from build123d import *

# Parameters (mm, degrees)
SKETCH1_W           = 50
SKETCH1_H           = 85
SKETCH1_R           = 1.25
BOSS_EXTRUDE3_DEPTH = 4
SKETCH2_W           = 50
SKETCH2_H           = 85
SKETCH2_W_2         = 47
SKETCH2_H_2         = 82
BOSS_EXTRUDE4_DEPTH = 25


with BuildPart() as part:
    # Sketch1 → Boss-Extrude3 (new body)
    with BuildSketch(Plane(origin=(0, 0, 0), x_dir=(1, 0, 0), z_dir=(0, 1, 0))):
        with Locations((23, 40.5)):
            Rectangle(SKETCH1_W, SKETCH1_H)
        with Locations((1.25, 79.75)):
            Circle(SKETCH1_R, mode=Mode.SUBTRACT)
        with Locations((44.75, 79.75)):
            Circle(SKETCH1_R, mode=Mode.SUBTRACT)
        with Locations((44.75, 1.25)):
            Circle(SKETCH1_R, mode=Mode.SUBTRACT)
        with Locations((1.25, 1.25)):
            Circle(SKETCH1_R, mode=Mode.SUBTRACT)
    extrude(amount=BOSS_EXTRUDE3_DEPTH)

    # Sketch2 → Boss-Extrude4 (add)
    with BuildSketch(Plane(origin=(0, 4, 0), x_dir=(1, 0, 0), z_dir=(0, 1, 0))):
        with Locations((23, 40.5)):
            Rectangle(SKETCH2_W, SKETCH2_H)
        with Locations((23, 40.5)):
            Rectangle(SKETCH2_W_2, SKETCH2_H_2, mode=Mode.SUBTRACT)
    extrude(amount=BOSS_EXTRUDE4_DEPTH)


solid = part.part
Source: CAD feature listing. Evaluate the final solid. Frame: model axes, mm. A direction names the side the tool comes from. Give positions to 0.01 mm unless a question says otherwise; leave off trailing zeros. Write each loop counter-clockwise with the first axis right and the second up, starting at its lowest first coordinate (ties: lowest second). Pieces come first, ordered by that corner, then holes. Notation, with made-up numbers: (22, 80.5) - (34, 80.5) arc R11 ccw to (34, 95.5) - close; hole circle Ø11 at (0.5, 18). An arc over 180 degrees is marked (long way). Write item = value, one per line. Start each with the question number.
Q1. Cut plane A-A, the plane z = -79.75. Return loops of the section in (x, y), then the cut area to 3 significant figures.
Q2. Material intervals for probe 1 along Z at (x, y) = (44.75, 1.2); probe 2 along X at (y, z) = (2.7, -79.75); probe 3 along Z at (x, y) = (9.5, 10.5), sorted ascending.
Q3. Draft query along Z for faces 3 (the cylindrical face through (0.26, 1.97, -0.49)), 4 (the flat face through (23, 0, -41)), 5 (the flat face through (23, 14, -83)). Return one class per face: +Z half, -Z half, draft (parallel to the pull), parting line (faces both ways), or undercut.
Q4. Pin query (flat end, axial travel): pin 1 Ø1.5 at (x, z) = (27, -70) entering from +Y; pin 2 Ø1.5 at (x, z) = (44.75, -79.75) entering from +Y. Return the tip coordinate at first contact, or that it passes through.
Q5. Reachability of faces 1 (the flat face through (-0.5, 16, -40)), 2 (the flat face through (-2, 14, -40)) from +Z, -Z, +X, -X, +Y, -Y: full face, straight path, thin tool, end or side. Return the list, or none.
Q6. Cut plane B-B, the plane y = 11.5. Return loops of the section in (x, z), then the cut area to 3 significant figures.
Q7. Cut plane C-C, the plane x = 44.75. Return loops of the section in (y, z).
Q8. Cut plane D-D, the plane x = 8.5. Return loops of the section in (y, z).
Computed values:
q1.outline = (-2, 0) - (0, 0) - (0, 4) - (-0.5, 4) - (-0.5, 29) - (-2, 29) - close; (2.5, 0) - (43.5, 0) - (43.5, 4) - (2.5, 4) - close; (46, 0) - (48, 0) - (48, 29) - (46.5, 29) - (46.5, 4) - (46, 4) - close
q1.area = 255 mm²
q2.probe_1 = -83 to -81, -78.5 to -2.5, 0 to 2
q2.probe_2 = -2 to 0, 2.5 to 43.5, 46 to 48
q2.probe_3 = -83 to -81.5, 0.5 to 2
q3.face_3 = undercut
q3.face_4 = draft
q3.face_5 = -Z half
q4.pin_1 = 4
q4.pin_2 = through
q5.face_1 = +Y
q5.face_2 = +Z, -Z, -X, +Y, -Y
q6.outline = (-2, -83) - (48, -83) - (48, 2) - (-2, 2) - close; hole (-0.5, -81.5) - (46.5, -81.5) - (46.5, 0.5) - (-0.5, 0.5) - close
q6.area = 396 mm²
q7.outline = (0, -83) - (29, -83) - (29, -81.5) - (4, -81.5) - (4, -81) - (0, -81) - close; (0, -78.5) - (4, -78.5) - (4, -2.5) - (0, -2.5) - close; (0, 0) - (4, 0) - (4, 0.5) - (29, 0.5) - (29, 2) - (0, 2) - close
q8.outline = (0, -83) - (29, -83) - (29, -81.5) - (4, -81.5) - (4, 0.5) - (29, 0.5) - (29, 2) - (0, 2) - close
